The listing builds one solid part. Answer for the finished solid, in the listing's coordinates (mm). Round coordinates to 2 decimals unless told otherwise and drop trailing zeros. Loops run counter-clockwise (first coordinate to the right, second up) from the corner with the lowest first, then second, coordinate; pieces in that order, holes last. Notation, with made-up numbers: (68.25, 19.5) -> (76.25, 19.5) arc R16 cw to (76.25, 32.5) -> close; hole circle Ø9 at (-33.5, 59). An arc over 180 degrees is marked (long way). Write each question's results on one line, items separated by ' | '. Start each with the question number.
(1) The part is cut by section B-B (x = 49). Determine the outline of the cut face in (y, z).
(2) The part is cut by section D-D (y = -5.75). Determine the outline of the cut face in (x, z), plus the area to 3 significant figures.
(3) The part is cut by section A-A (y = 0). Determine the outline of the cut face in (x, z), plus the area to 3 significant figures.
(4) Straight lines are drawn through the part: probe 1 along Y at (x, z) = (-49, 5.2); probe 2 along X at (y, z) = (-1.75, 4.25); probe 3 along X at (y, z) = (-2.25, 2). For each, find the intervals that lie inside material, in ascending order.
(5) The part is cut by section C-C (z = 1.5). Determine the outline of the cut face in (x, y).
(6) Flat-ended cylindrical pins translate along their axes: pin 1 (0.7 mm diameter, centred on y = 2.5, z = 2, fed in from +X); pin 2 (1.1 mm diameter, centred on y = -0.5, z = 2, fed in from -X); pin 3 (4 mm diameter, centred on x = 49, y = 0, fed in from -Z); pin 4 (7.5 mm diameter, centred on x = -43.5, y = -1, fed in from -Z). Find the tip coordinate at first contact, or state that the pin passes through.
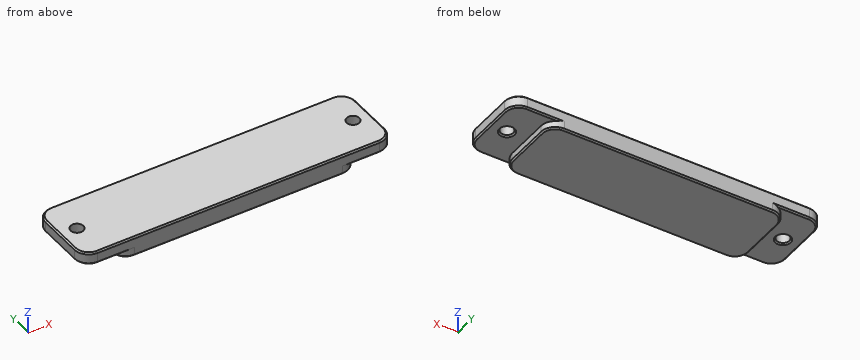
```python
from build123d import *

# Parameters (mm, degrees)
F1_DEPTH = 2.7
F3_R     = 2.25
F4_DEPTH = 4.3
F5_SIZE  = 0.5


with BuildPart() as f1:
    # F0 (on Top) → F1 (new body)
    with BuildSketch(Plane.XY):
        with BuildLine():
            Line((37, 13), (-37, 13))
            ThreePointArc((-37, 13), (-40.535534, 11.535534), (-42, 8))
            Line((-42, 8), (-42, -8))
            ThreePointArc((-42, -8), (-40.535534, -11.535534), (-37, -13))
            Line((-37, -13), (37, -13))
            ThreePointArc((37, -13), (40.535534, -11.535534), (42, -8))
            Line((42, -8), (42, 8))
            ThreePointArc((42, 8), (40.535534, 11.535534), (37, 13))
        make_face()
    extrude(amount=F1_DEPTH)

    # F3 (on face) → F4 (join, through all)
    with BuildSketch(Plane.XY.offset(2.7)):
        with BuildLine():
            Line((37, 13), (-37, 13))
            ThreePointArc((-37, 13), (-40.535534, 11.535534), (-42, 8))
            Line((-42, 8), (-42, -8))
            ThreePointArc((-42, -8), (-40.535534, -11.535534), (-37, -13))
            Line((-37, -13), (37, -13))
            ThreePointArc((37, -13), (40.535534, -11.535534), (42, -8))
            Line((42, -8), (42, 8))
            ThreePointArc((42, 8), (40.535534, 11.535534), (37, 13))
        make_face()
        with BuildLine():
            Line((50, 13), (37, 13))
            ThreePointArc((37, 13), (40.535534, 11.535534), (42, 8))
            Line((42, 8), (42, -8))
            ThreePointArc((42, -8), (40.535534, -11.535534), (37, -13))
            Line((37, -13), (50, -13))
            ThreePointArc((50, -13), (53.535534, -11.535534), (55, -8))
            Line((55, -8), (55, 8))
            ThreePointArc((55, 8), (53.535534, 11.535534), (50, 13))
        make_face()
        with Locations((49, 0)):
            Circle(F3_R, mode=Mode.SUBTRACT)
        with BuildLine():
            Line((-37, 13), (-50, 13))
            ThreePointArc((-50, 13), (-53.535534, 11.535534), (-55, 8))
            Line((-55, 8), (-55, -8))
            ThreePointArc((-55, -8), (-53.535534, -11.535534), (-50, -13))
            Line((-50, -13), (-37, -13))
            ThreePointArc((-37, -13), (-40.535534, -11.535534), (-42, -8))
            Line((-42, -8), (-42, 8))
            ThreePointArc((-42, 8), (-40.535534, 11.535534), (-37, 13))
        make_face()
        with Locations((-49, 0)):
            Circle(F3_R, mode=Mode.SUBTRACT)
    extrude(amount=F4_DEPTH)

    # F5
    f5_edges = [f1.edges().sort_by_distance(p)[0] for p in [
        (0, -13, 0),
        (46.75, 0, 2.7),
        (-51.25, 0, 2.7),
        (43.5, 13, 2.7),
        (-43.5, 13, 2.7),
        (0, 13, 7),
    ]]
    chamfer(f5_edges, length=F5_SIZE)


solid = f1.part
```
Checked values:
1) outline: (-13, 3.2) -> (-12.5, 2.7) -> (-2.75, 2.7) -> (-2.25, 3.2) -> (-2.25, 7) -> (-12.5, 7) -> (-13, 6.5) -> close; (2.25, 3.2) -> (2.75, 2.7) -> (12.5, 2.7) -> (13, 3.2) -> (13, 6.5) -> (12.5, 7) -> (2.25, 7) -> close
2) outline: (-55, 3.2) -> (-54.5, 2.7) -> (-42, 2.7) -> (-42, 0.5) -> (-41.5, 0) -> (41.5, 0) -> (42, 0.5) -> (42, 2.7) -> (54.5, 2.7) -> (55, 3.2) -> (55, 6.5) -> (54.5, 7) -> (-54.5, 7) -> (-55, 6.5) -> close | area: 699 mm2
3) outline: (-55, 3.2) -> (-54.5, 2.7) -> (-51.75, 2.7) -> (-51.25, 3.2) -> (-51.25, 7) -> (-54.5, 7) -> (-55, 6.5) -> close; (-46.75, 3.2) -> (-46.25, 2.7) -> (-42, 2.7) -> (-42, 0.5) -> (-41.5, 0) -> (41.5, 0) -> (42, 0.5) -> (42, 2.7) -> (46.25, 2.7) -> (46.75, 3.2) -> (46.75, 7) -> (-46.75, 7) -> close; (51.25, 3.2) -> (51.75, 2.7) -> (54.5, 2.7) -> (55, 3.2) -> (55, 6.5) -> (54.5, 7) -> (51.25, 7) -> close | area: 660 mm2
4) probe 1: y = -13 to -2.25, 2.25 to 13 | probe 2: x = -55 to -50.41, -47.59 to 47.59, 50.41 to 55 | probe 3: x = -42 to 42
5) outline: (-42, -8) arc R5 ccw to (-37, -13) -> (37, -13) arc R5 ccw to (42, -8) -> (42, 8) arc R5 ccw to (37, 13) -> (-37, 13) arc R5 ccw to (-42, 8) -> close
6) pin 1: stops at x = 42 | pin 2: stops at x = -42 | pin 3: passes through | pin 4: stops at z = 0
